Check sheet for the modelled part. Datum: model origin and axes. Units: mm. Face numbers are marked on the shaded views. A direction names the side the tool comes from. Round coordinates to 2 decimals unless told otherwise and drop trailing zeros. Loops run counter-clockwise (first coordinate to the right, second up) from the corner with the lowest first, then second, coordinate; pieces in that order, holes last. Notation, with made-up numbers: (65.5, 6.25) - (107.5, 6.25) arc R30 ccw to (107.5, 33.25) - close; hole circle Ø1 at (18.5, 61.25). An arc over 180 degrees is marked (long way). Put each result on its own line as item: value. Start each with the question number.
```python
from build123d import *

# Parameters (mm, degrees)
BODY_DEPTH          = 38
SHELL1_START        = -36
SHELL1_DEPTH        = 72
HOLE_DEPTH          = 41.471872949
HOLE_DEPTH_BACK     = 41.471872949
SKETCH2_W           = 20
SKETCH2_H           = 5
SKETCH3_R           = 1.75
FIXATION_HOLE_DEPTH = 43.660754799


# Read off the part's stored shape, not the designer's step: Shell1
with BuildPart() as part:
    # Sketch1 → Body (new, symmetric)
    with BuildSketch(Plane(origin=(0, 0, 0), x_dir=(0, 0, -1), z_dir=(1, 0, 0))):
        with BuildLine():
            Line((10.5, -9.15), (-10.5, -9.15))
            Line((-10.5, -9.15), (-10.5, 4.15))
            ThreePointArc((-10.5, 4.15), (-9.035533906, 7.685533906), (-5.5, 9.15))
            Line((-5.5, 9.15), (5.5, 9.15))
            ThreePointArc((5.5, 9.15), (9.035533906, 7.685533906), (10.5, 4.15))
            Line((10.5, 4.15), (10.5, -9.15))
        make_face()
    extrude(amount=BODY_DEPTH, both=True)

    # Shell1 outline → Shell1 (cut)
    with BuildSketch(Plane.YZ.offset(SHELL1_START)):
        with BuildLine():
            Line((7.15, -5.5), (9.15, -5.5))
            Line((9.15, -5.5), (9.15, 5.5))
            Line((9.15, 5.5), (7.15, 5.5))
            ThreePointArc((7.15, 5.5), (6.271320344, 7.621320344), (4.15, 8.5))
            Line((4.15, 8.5), (-7.15, 8.5))
            Line((-7.15, 8.5), (-7.15, -8.5))
            Line((-7.15, -8.5), (4.15, -8.5))
            ThreePointArc((4.15, -8.5), (6.271320344, -7.621320344), (7.15, -5.5))
        make_face()
    extrude(amount=SHELL1_DEPTH, mode=Mode.SUBTRACT)

    # Sketch2 → Hole (cut, two sides: drawn at the far end of the back side and taken through both)
    with BuildSketch(Plane.XY.offset(-HOLE_DEPTH_BACK)):
        with Locations((0, 6.65)):
            Rectangle(SKETCH2_W, SKETCH2_H)
    extrude(amount=HOLE_DEPTH + HOLE_DEPTH_BACK, mode=Mode.SUBTRACT)

    # Sketch3 → Fixation_Hole (cut, through all)
    with BuildSketch(Plane(origin=(0, -7.15, 0), x_dir=(1, 0, 0), z_dir=(0, 1, 0))):
        with Locations(Location((0, 0, 0), (0, 0, 270))):
            Circle(SKETCH3_R)
    extrude(amount=-FIXATION_HOLE_DEPTH, mode=Mode.SUBTRACT)


solid = part.part
```
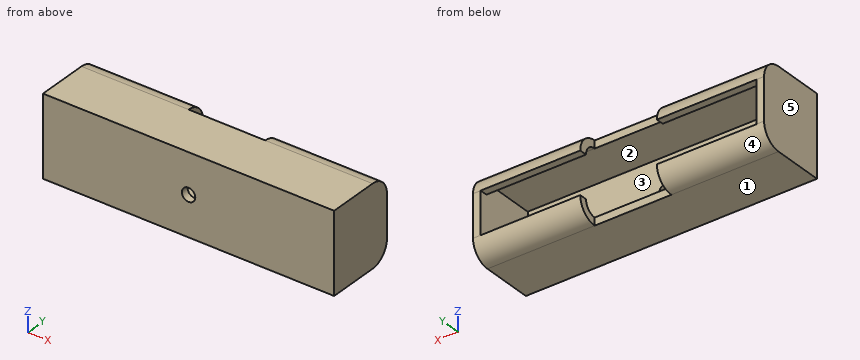
Q1. Depth check by flat-ended pin: pin 1 Ø2 at (x, y) = (21, 8.5) entering from +Z; pin 2 Ø1.6 at (x, y) = (-19, 8) entering from -Z; pin 3 Ø3 at (x, z) = (0, 0) entering from +Y; pin 4 Ø2 at (x, z) = (-1.5, -9.5) entering from +Y. Enter the tip coordinate at first touch or a pass-through.
Q2. Cross-section at C-C on y = 1. Enter the section's corners in (x, z).
Q3. Draft check along X on the marked faces 3, 4 and 5. Enter one of: +X half, -X half, draft (parallel to the pull), parting line (faces both ways), or undercut.
Q4. Material ranges on line 1 (X direction, y = -7.55, z = 0); line 2 (Z direction, x = -34, y = -4.5); line 3 (X direction, y = -6.25, z = -8), recorded low to high. Write a range as from..to.
Q5. Cross-section at D-D on z = 4.5. Enter the section's corners in (x, y), and give its area (3 significant figures).
Q6. Set-up check for the marked faces 1 and 2: record each of +Z, -Z, +X, -X, +Y, -Y from which the full face is reachable in a straight line by a thin tool's end or side.
Q7. Cross-section at B-B on x = 0. Enter the section's corners in (y, z), and give its area (3 significant figures).
Q8. Cross-section at A-A on z = 0. Enter the section's corners in (x, y).
Answer list:
1. pin 1: stops at z = 9.21
1. pin 2: stops at z = -9.46
1. pin 3: passes through
1. pin 4: stops at y = 4.15
2. outline: (-38, -10.5) - (38, -10.5) - (38, 10.5) - (-38, 10.5) - close; hole (-36, -8.5) - (36, -8.5) - (36, 8.5) - (-36, 8.5) - close
3. face 3: undercut
3. face 4: draft
3. face 5: -X half
4. line 1: x = -38..-1.75, 1.75..38
4. line 2: z = -10.5..-8.5, 8.5..10.5
4. line 3: x = -38..-36, 36..38
5. outline: (-38, -9.15) - (38, -9.15) - (38, 9.15) - (36, 9.15) - (36, -7.15) - (-36, -7.15) - (-36, 9.15) - (-38, 9.15) - close
5. area: 217 mm2
6. face 1: -Z, +X, -X, +Y, -Y
6. face 2: none
7. outline: (-9.15, -10.5) - (4.15, -10.5) - (4.15, -8.5) - (-7.15, -8.5) - (-7.15, -1.75) - (-9.15, -1.75) - close; (-9.15, 1.75) - (-7.15, 1.75) - (-7.15, 8.5) - (4.15, 8.5) - (4.15, 10.5) - (-9.15, 10.5) - close
7. area: 80.2 mm2
8. outline: (-38, -9.15) - (-1.75, -9.15) - (-1.75, -7.15) - (-36, -7.15) - (-36, 9.15) - (-38, 9.15) - close; (1.75, -9.15) - (38, -9.15) - (38, 9.15) - (36, 9.15) - (36, -7.15) - (1.75, -7.15) - close
